Source: CAD feature listing. Evaluate the final solid. Frame: model axes, mm. Coordinates: 2 decimals unless noted, no trailing zeros. Loops run counter-clockwise (first coordinate to the right, second up) from the corner with the lowest first, then second, coordinate; pieces in that order, holes last.
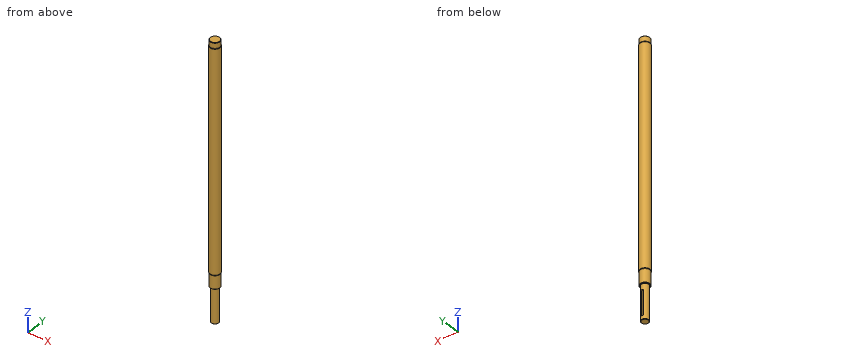
Autodesk Inventor part; units mm, degrees
ref_plane "Work Plane1" through (0, 9, -352.5) normal (0, 1, 0) x (-1, 0, 0)
ref_plane "YZ Plane" through (0, 0, 0) normal (1, 0, 0) x (0, 1, 0)
ref_plane "XY Plane" through (0, 0, 0) normal (0, 0, 1) x (1, 0, 0)
sketch "Sketch1" plane through (0, 0, 0) normal (0, 1, 0) x (-1, 0, 0)
  line L0 (0, 0) -> (0, 280)
  line L1 (0, 280) -> (-12.5, 280)
  line L2 (-12.5, 280) -> (-12.5, 0)
  line L3 (-12.5, 0) -> (-12.5, -395)
  line L4 (-12.5, -395) -> (0, -395)
  line L5 (0, -395) -> (0, 0)
  line L6 (-9, -395) -> (-9, -310)
  line L7 (-9, -310) -> (-12.5, -310)
  line L8 (-12.5, -275) -> (-12, -275)
  line L9 (-12, -275) -> (-12, -310)
  line L10 (-12, 280) -> (-12, 265)
  line L11 (-12, 265) -> (-12.5, 265)
  line L12 (-12, 265) -> (-11, 265)
  line L13 (-11, 265) -> (-11, 267)
  line L14 (-11, 267) -> (-12, 267)
  line L15 (-12, -275) -> (-11, -275)
  line L16 (-11, -275) -> (-11, -277)
  line L17 (-11, -277) -> (-12, -277)
  dimension "d0" = 25
  dimension "d1" = 280
  dimension "d2" = 395
  dimension "d4" = 85
  dimension "d5" = 18
  dimension "d6" = 24
  dimension "d7" = 35
  dimension "d8" = 15
  dimension "d18" = 22
  dimension "d19" = 2
revolve "Revolution1" add sketch "Sketch1" angle 360 about axis through (0, 0, 0) along (0, 0, 1) contours L5 L4 L6 L7 L9 L17 L16 L15 L8 L3 L2 L11 L12 L13 L14 L10 L1 L0
ref_plane "Work Plane1" through (0, 9, -352.5) normal (0, 1, 0) x (-1, 0, 0)
sketch "Sketch2" plane through (0, 9, -352.5) normal (0, 1, 0) x (-1, 0, 0)
  line L0 (9, -42.5) -> (-9, -42.5)
  line L1 (9, 42.5) -> (-9, 42.5)
  line L2 (9, -42.5) -> (9, 42.5)
  line L3 (-9, -42.5) -> (-9, 42.5)
  line L4 (9, -40.905) -> (-9, -40.905) construction
  line L5 (9, 37.095) -> (-9, 37.095) construction
  line L6 (0, 29.595) -> (0, -33.405) construction
  line L7 (-3, 26.595) -> (-3, -30.405)
  line L8 (3, -30.405) -> (3, 26.595)
  arc A0 (3, 26.595) -> (-3, 26.595) centre (0, 26.595) ccw
  arc A1 (-3, -30.405) -> (3, -30.405) centre (0, -30.405) ccw
  line L9 (0, 37.095) -> (0, -40.905) construction
  point P0 (0, 352.5)
  point P1 (0, -1.905)
  point P2 (0, -1.905)
  dimension "d9" = 1.595
  dimension "d10" = 78
  dimension "d11" = 63
  dimension "d12" = 6
extrude "Extrusion1" cut sketch "Sketch2" against normal blind 3.5 contours A0 L8 A1 L7
chamfer "Chamfer1" distance 1 angle 45 3 edges at (-9, 0, -395) (-12, 0, 280) (-12, 0, -310)
properties part number "TRM 028 main shaft"
Q1. Line query: line 1 along Z through (x, y) = (-11, 1.5); line 2 along Z through (x, y) = (-7.5, -9); line 3 along X through (y, z) = (-3.5, -204). Output: solid intervals per line, ascending.
Q2. Contact query for flat-ended pins moving along their axis: pin 1 Ø3.5 at (y, z) = (7.5, -363.5) entering from +X; pin 2 Ø12 at (y, z) = (6, -318) entering from +X; pin 3 Ø1.5 at (x, z) = (-3.5, -321) entering from -Y; pin 4 Ø10 at (x, z) = (5, -262) entering from +Y. Output: stop coordinate, or through.
Q3. Section B-B, the plane z = -143. Return the cut outline in (x, y).
Derived:
1. line 1: z = -309.9 to -277, -275 to 265, 267 to 279.9
1. line 2: z = -309.28 to -277, -275 to 265, 267 to 279.28
1. line 3: x = -12 to 12
2. pin 1: stops at x = 6.92
2. pin 2: stops at x = 9
2. pin 3: stops at y = -8.57
2. pin 4: stops at y = 12.5
3. outline: circle Ø25 at (0, 0)
